Verification items for the finished model (mm, model axes). A direction names the side the tool comes from. Give positions to 0.01 mm unless a question says otherwise; leave off trailing zeros. Write each loop counter-clockwise with the first axis right and the second up, starting at its lowest first coordinate (ties: lowest second). Pieces come first, ordered by that corner, then holes. Notation, with made-up numbers: (36.25, -38.75) - (68.25, -38.75) arc R18 cw to (68.25, -19.75) - close; hole circle Ø3 at (49, 89.25). An arc over 180 degrees is marked (long way). Put each result on its own line as item: value.
from build123d import *

# Parameters (mm, degrees)
BOSS_EXTRUDE1_DEPTH = 3.175


with BuildPart() as part:
    # Sketch2 → Boss-Extrude1 (new body)
    with BuildSketch(Plane(origin=(0, 0, 0), x_dir=(1, 0, 0), z_dir=(0, 1, 0))):
        Polygon((-152.4, 116.478975516), (-116.478975516, 152.4), (116.478975516, 152.4), (152.4, 116.478975516), (152.4, -116.478975516), (116.478975516, -152.4), (-116.478975516, -152.4), (-152.4, -116.478975516), align=None)
        with BuildLine():
            Line((-116.478975516, 80.557951031), (-80.557951031, 116.478975516))
            Line((-80.557951031, 116.478975516), (-80.557951031, 120.65))
            ThreePointArc((-80.557951031, 120.65), (-76.838207153, 129.630256121), (-67.857951031, 133.35))
            Line((-67.857951031, 133.35), (67.857951031, 133.35))
            ThreePointArc((67.857951031, 133.35), (76.838207153, 129.630256121), (80.557951031, 120.65))
            Line((80.557951031, 120.65), (80.557951031, 116.478975516))
            Line((80.557951031, 116.478975516), (116.478975516, 80.557951031))
            Line((116.478975516, 80.557951031), (120.65, 80.557951031))
            ThreePointArc((120.65, 80.557951031), (129.630256121, 76.838207153), (133.35, 67.857951031))
            Line((133.35, 67.857951031), (133.35, -67.857951031))
            ThreePointArc((133.35, -67.857951031), (129.630256121, -76.838207153), (120.65, -80.557951031))
            Line((120.65, -80.557951031), (116.478975516, -80.557951031))
            Line((116.478975516, -80.557951031), (80.557951031, -116.478975516))
            Line((80.557951031, -116.478975516), (80.557951031, -120.65))
            ThreePointArc((80.557951031, -120.65), (76.838207153, -129.630256121), (67.857951031, -133.35))
            Line((67.857951031, -133.35), (-67.857951031, -133.35))
            ThreePointArc((-67.857951031, -133.35), (-76.838207153, -129.630256121), (-80.557951031, -120.65))
            Line((-80.557951031, -120.65), (-80.557951031, -116.478975516))
            Line((-80.557951031, -116.478975516), (-116.478975516, -80.557951031))
            Line((-116.478975516, -80.557951031), (-120.65, -80.557951031))
            ThreePointArc((-120.65, -80.557951031), (-129.630256121, -76.838207153), (-133.35, -67.857951031))
            Line((-133.35, -67.857951031), (-133.35, 67.857951031))
            ThreePointArc((-133.35, 67.857951031), (-129.630256121, 76.838207153), (-120.65, 80.557951031))
            Line((-120.65, 80.557951031), (-116.478975516, 80.557951031))
        make_face(mode=Mode.SUBTRACT)
    extrude(amount=BOSS_EXTRUDE1_DEPTH)


solid = part.part
Q1. Section check C-C, the plane z = -6.5. Record the cut outline in (x, y) (3 decimals), plus the area to 3 significant figures.
Answers follow:
outline: (-152.4, 0) - (-133.35, 0) - (-133.35, 3.175) - (-152.4, 3.175) - close; (133.35, 0) - (152.4, 0) - (152.4, 3.175) - (133.35, 3.175) - close
area: 121 mm2
Q2. Section check B-B, the plane x = 13.5. Record the cut outline in (y, z) (3 decimals).
Answers follow:
outline: (0, -152.4) - (3.175, -152.4) - (3.175, -133.35) - (0, -133.35) - close; (0, 133.35) - (3.175, 133.35) - (3.175, 152.4) - (0, 152.4) - close
Q3. Set-up check for faces 4 (the face through (-134.69, 1.57, -134.19)), 5 (the face through (76.74, 1.57, -129.73)): record each of +Z, -Z, +X, -X, +Y, -Y from which the full face is reachable in a straight line by a thin tool's end or side.
Answers follow:
face 4: -Z, -X, +Y, -Y
face 5: +Y, -Y
Q4. Scan lines: line 1 along X through (y, z) = (2.6, 36); line 2 along Z through (x, y) = (-120, 2.4). Record each from-to range of solid material in increasing order.
Answers follow:
line 1: x = -152.4 to -133.35, 133.35 to 152.4
line 2: z = -148.88 to -80.56, 80.56 to 148.88
Q5. Release check for a two-part mould opening along X. For faces 1 (the face through (134.19, 1.57, -134.69)), 2 (the face through (1, 0, -136)), 3 (the face through (-76.74, 1.57, 129.73)) record: released by +X, released by -X, zero draft, split by the parting line, or undercut.
Answers follow:
face 1: released by +X
face 2: zero draft
face 3: undercut
Q6. Go/stop test with flat-tipped pins: pin 1 Ø1.6 at (x, y) = (118, 2) entering from -Z; pin 2 Ø1.6 at (y, z) = (1, -118) entering from +X; pin 3 Ø1 at (y, z) = (2, 119) entering from +X. Record where each tip stops, or that it passes through.
Answers follow:
pin 1: stops at z = -151.68
pin 2: stops at x = 151.68
pin 3: stops at x = 150.38
